The figure shows three views and two pictorial views of one solid part (mm, origin at its lowest corner). Answer the questions. A direction names the side the tool comes from. Coordinates: 2 decimals unless noted, no trailing zeros. Loops run counter-clockwise (first coordinate to the right, second up) from the corner with the lowest first, then second, coordinate; pieces in that order, holes last. Notation, with made-up numbers: (0.5, 57) - (40.5, 57) arc R18 ccw to (40.5, 78) - close; hole circle Ø10 at (54, -16). An arc over 180 degrees is marked (long way). One line per question, with ' | ' between items.
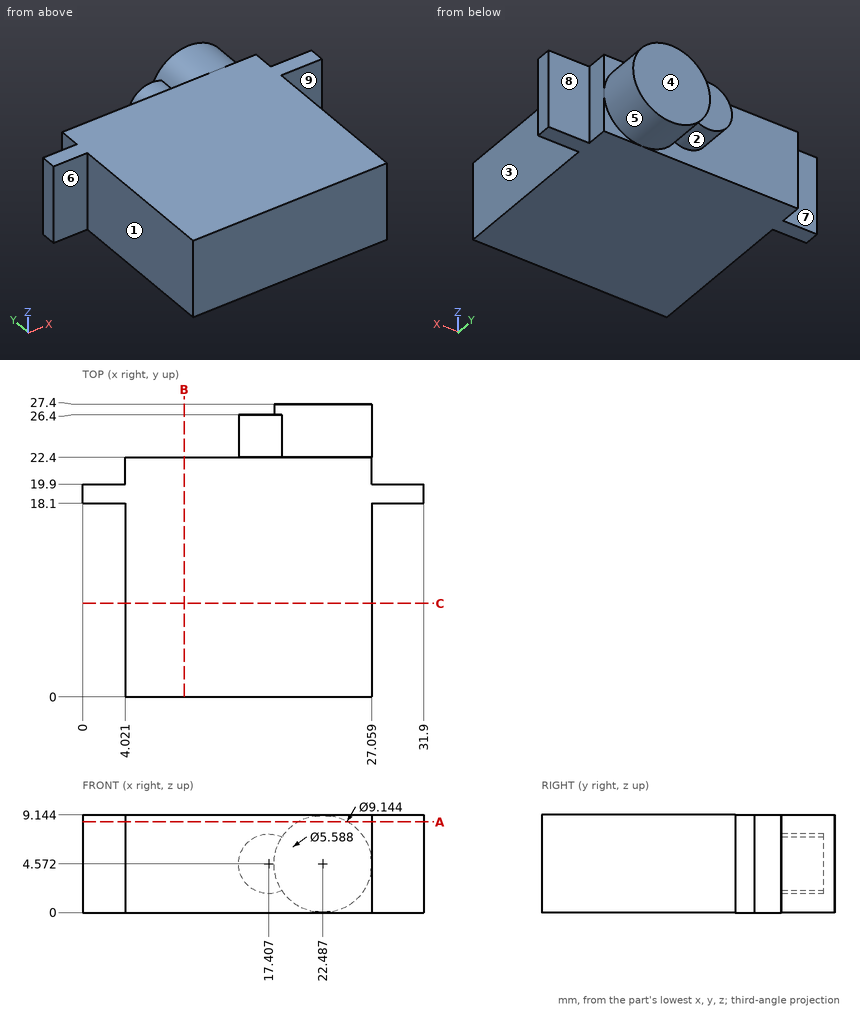
Item 1: Which of the six approach directions +Z, -Z, +X, -X, +Y, -Y give full straight-line access (tool end or side, diameter ignored) to the marked faces 5, 6, 7, 8 and 9?
Taken from the geometry:
face 5: +Y | face 6: +Z, -Z, -X, -Y | face 7: +Z, -Z, -X, +Y | face 8: +Z, -Z, +X, +Y | face 9: +Z, -Z, +X, -Y
Item 2: The mould has two halves that part along X. Classify the marked faces 1, 2, 3 and 4: pulls with the +X half, pulls with the -X half, needs draft (parallel to the pull), parting line crosses it, or undercut.
Taken from the geometry:
face 1: pulls with the -X half | face 2: undercut | face 3: pulls with the +X half | face 4: needs draft
Item 3: Find section B-B, the plane x = 9.5. Write down the section's boundary in (y, z), plus the area to 3 significant figures.
Taken from the geometry:
outline: (0, 0) - (22.4, 0) - (22.4, 9.14) - (0, 9.14) - close | area: 205 mm2
Item 4: Each of these flat-tipped pins is pushed along its axis until it touches: pin 1 Ø2 at (y, z) = (21, 5) entering from +X; pin 2 Ø2.5 at (x, z) = (29, 2.5) entering from +Y; pin 3 Ø4.5 at (x, z) = (16.5, 5) entering from +Y; pin 4 Ø4 at (x, z) = (4, 6.5) entering from +Y. Where does it stop, or does it pass through?
Taken from the geometry:
pin 1: stops at x = 27.06 | pin 2: stops at y = 19.9 | pin 3: stops at y = 27.4 | pin 4: stops at y = 22.4
Item 5: Find section A-A, the plane z = 8.5. Write down the section's boundary in (x, y).
Taken from the geometry:
outline: (0, 18.1) - (4.02, 18.1) - (4.02, 0) - (27.06, 0) - (27.06, 18.1) - (31.9, 18.1) - (31.9, 19.9) - (27.06, 19.9) - (27.06, 22.4) - (24.83, 22.4) - (24.83, 27.4) - (20.15, 27.4) - (20.15, 22.4) - (4.02, 22.4) - (4.02, 19.9) - (0, 19.9) - close
Item 6: Find the intervals of material crossed by line 1 (X direction, y = 13.75, z = 3.5); line 2 (Y direction, x = 13, z = 5); line 3 (Y direction, x = 17.5, z = 5.5), in increasing order. Write a range as [from, to].
Taken from the geometry:
line 1: x = [4.02, 27.06] | line 2: y = [0, 22.4] | line 3: y = [0, 26.4]
Item 7: Find section C-C, the plane y = 8.75. Write down the section's boundary in (x, z), plus the area to 3 significant figures.
Taken from the geometry:
outline: (4.02, 0) - (27.06, 0) - (27.06, 9.14) - (4.02, 9.14) - close | area: 211 mm2
